Design review of the part built by this model. Coordinates are the model's own, in mm. Face numbers are marked on the shaded views. Coordinates: 2 decimals unless noted, no trailing zeros. Write each loop counter-clockwise with the first axis right and the second up, starting at its lowest first coordinate (ties: lowest second). Pieces come first, ordered by that corner, then holes. Notation, with made-up numbers: (88.5, 18.5) -> (93.5, 18.5) arc R26 ccw to (93.5, 52.5) -> close; hole circle Ø2 at (25.5, 41). An arc over 180 degrees is marked (long way). Answer in a Markdown table with one row per item. Add a question column.
Item 1: Draft analysis for pull direction Y (two halves, no side actions). For the marked faces 1, 2 and 3, state which applies: released by +Y, released by -Y, zero draft, split by the parting line, or undercut.
Item 2: Take a section at C-C, the plane y = -2.75. Write out the cut boundary in (x, z), and give its area (3 significant figures).
Item 3: Clearance check with a flat-ended pin moving along its axis: P1, Ø4, axis at x = 9, y = 0, coming from the -Z side. State where the tip first meets the part, or that it passes through.
Item 4: To check wall thickness, follow line 1 (Y direction, x = 2, z = 1.5); line 2 (Z direction, x = -17.5, y = 1.25); line 3 (X direction, y = 0.5, z = 2.5). State the ranges of each line that lie inside material, in increasing order.
Item 5: Take a section at A-A, the plane z = 5.75. Write out the cut boundary in (x, y).
Item 6: Take a section at B-B, the plane x = -16. Write out the cut boundary in (y, z), and give its area (3 significant figures).
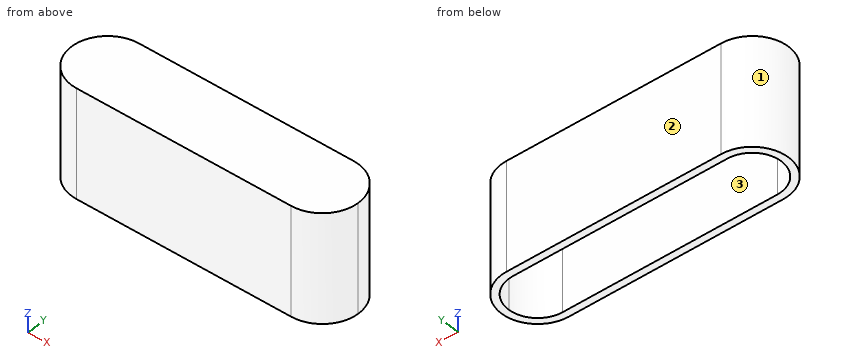
from build123d import *

# Parameters (mm, degrees)
F1_DEPTH = 15
F3_DEPTH = 10


with BuildPart() as f1:
    # F0 (on Top) → F1 (new body)
    with BuildSketch(Plane.XY):
        with BuildLine():
            ThreePointArc((15, 5), (10, 0), (15, -5))
            Line((15, -5), (15, 5))
        make_face()
        with BuildLine():
            Line((-15, -5), (15, -5))
            ThreePointArc((15, -5), (10, 0), (15, 5))
            Line((15, 5), (-15, 5))
            ThreePointArc((-15, 5), (-11.4644660941, 3.5355339059), (-10, 0))
            ThreePointArc((-10, 0), (-11.4644660941, -3.5355339059), (-15, -5))
        make_face()
        with BuildLine():
            Line((15, 5), (15, -5))
            ThreePointArc((15, -5), (18.5355339059, -3.5355339059), (20, 0))
            ThreePointArc((20, 0), (18.5355339059, 3.5355339059), (15, 5))
        make_face()
        with BuildLine():
            ThreePointArc((-15, 5), (-20, 0), (-15, -5))
            Line((-15, -5), (-15, 5))
        make_face()
        with BuildLine():
            Line((-15, 5), (-15, -5))
            ThreePointArc((-15, -5), (-11.4644660941, -3.5355339059), (-10, 0))
            ThreePointArc((-10, 0), (-11.4644660941, 3.5355339059), (-15, 5))
        make_face()
    extrude(amount=F1_DEPTH)

    # F2 (on face) → F3 (cut)
    with BuildSketch(Plane(origin=(0, 0, 0), x_dir=(1, 0, 0), z_dir=(0, 0, -1))):
        with BuildLine():
            ThreePointArc((15, 4), (11, 0), (15, -4))
            Line((15, -4), (15, 4))
        make_face()
        with BuildLine():
            Line((-15, -4), (15, -4))
            ThreePointArc((15, -4), (11, 0), (15, 4))
            Line((15, 4), (-15, 4))
            ThreePointArc((-15, 4), (-12.1715728753, 2.8284271247), (-11, 0))
            ThreePointArc((-11, 0), (-12.1715728753, -2.8284271247), (-15, -4))
        make_face()
        with BuildLine():
            Line((15, 4), (15, -4))
            ThreePointArc((15, -4), (17.8284271247, -2.8284271247), (19, 0))
            ThreePointArc((19, 0), (17.8284271247, 2.8284271247), (15, 4))
        make_face()
        with BuildLine():
            ThreePointArc((-15, 4), (-19, 0), (-15, -4))
            Line((-15, -4), (-15, 4))
        make_face()
        with BuildLine():
            Line((-15, 4), (-15, -4))
            ThreePointArc((-15, -4), (-12.1715728753, -2.8284271247), (-11, 0))
            ThreePointArc((-11, 0), (-12.1715728753, 2.8284271247), (-15, 4))
        make_face()
    extrude(amount=-F3_DEPTH, mode=Mode.SUBTRACT)


solid = f1.part
Answers:
| question | item | result |
|---|---|---|
| 1 | face 1 | split by the parting line |
| 1 | face 2 | released by +Y |
| 1 | face 3 | undercut |
| 2 | outline | (-19.18, 0) -> (-17.9, 0) -> (-17.9, 10) -> (17.9, 10) -> (17.9, 0) -> (19.18, 0) -> (19.18, 15) -> (-19.18, 15) -> close |
| 2 | area | 217 mm^2 |
| 3 | P1 | stops at z = 10 |
| 4 | line 1 | y = -5 to -4, 4 to 5 |
| 4 | line 2 | z = 10 to 15 |
| 4 | line 3 | x = -19.97 to -18.97, 18.97 to 19.97 |
| 5 | outline | (-15, -5) -> (15, -5) arc R5 ccw to (15, 5) -> (-15, 5) arc R5 ccw to start; hole (-15, -4) -> (15, -4) arc R4 ccw to (15, 4) -> (-15, 4) arc R4 ccw to start |
| 6 | outline | (-4.9, 0) -> (-3.87, 0) -> (-3.87, 10) -> (3.87, 10) -> (3.87, 0) -> (4.9, 0) -> (4.9, 15) -> (-4.9, 15) -> close |
| 6 | area | 69.5 mm^2 |
